Could you check a few things on this drawing? It's one solid part, dimensions in mm from its lowest x, y, z. Give positions to 0.01 mm unless a question says otherwise; leave off trailing zeros. Loops run counter-clockwise (first coordinate to the right, second up) from the corner with the lowest first, then second, coordinate; pieces in that order, holes last. Notation, with made-up numbers: (84.25, 45.25) - (121.25, 45.25) arc R21 cw to (121.25, 55.25) - close; hole circle Ø4 at (28, 56). An arc over 180 degrees is marked (long way). Use a Markdown table: item, result.
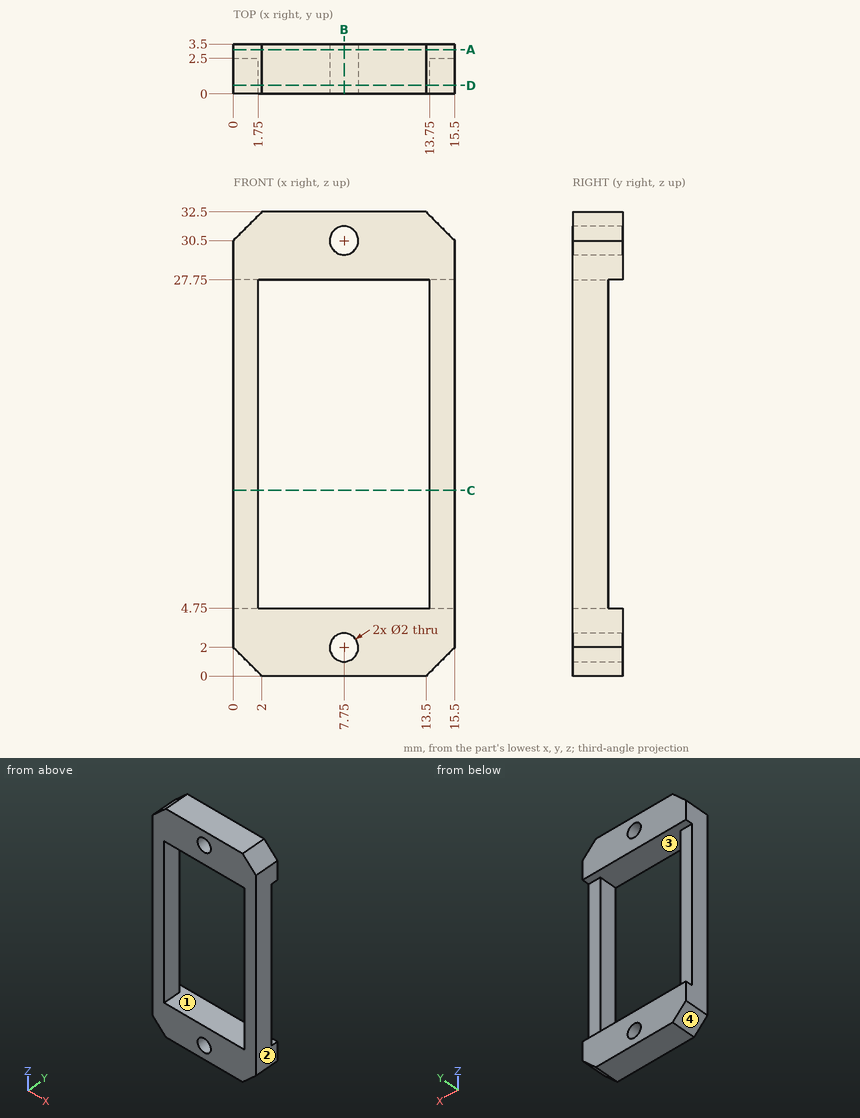
(1) Suppose I cut it at A-A on y = 3.1. Write out the boundary of the cut face in (x, z), plus the area to 3 significant figures.
A:
| item | result |
|---|---|
| outline | (0, 2) - (2, 0) - (13.5, 0) - (15.5, 2) - (15.5, 4.75) - (0, 4.75) - close; (0, 27.75) - (15.5, 27.75) - (15.5, 30.5) - (13.5, 32.5) - (2, 32.5) - (0, 30.5) - close; hole circle Ø2 at (7.75, 2); hole circle Ø2 at (7.75, 30.5) |
| area | 133 mm2 |
(2) We'd pull the mould along Z, two halves only. Please class the marked faces 1, 2, 3 and 4: pulls with the +Z half, pulls with the -Z half, needs draft (parallel to the pull), parting line crosses it, or undercut.
A:
| item | result |
|---|---|
| face 1 | undercut |
| face 2 | needs draft |
| face 3 | undercut |
| face 4 | pulls with the -Z half |
(3) If I drill on line 1 (Z direction, x = 3.75, y = 2.7); line 2 (X direction, y = 2.5, z = 30.5); line 3 (X direction, y = 1.5, z = 20), over which ranges is the centre line in solid material (lowest first)?
A:
| item | result |
|---|---|
| line 1 | 0 to 4.75, 27.75 to 32.5 |
| line 2 | 0 to 6.75, 8.75 to 15.5 |
| line 3 | 0 to 1.75, 13.75 to 15.5 |
(4) Suppose I cut it at C-C on z = 13. Write out the boundary of the cut face in (x, y).
A:
| item | result |
|---|---|
| outline | (0, 0) - (1.75, 0) - (1.75, 2.5) - (0, 2.5) - close; (13.75, 0) - (15.5, 0) - (15.5, 2.5) - (13.75, 2.5) - close |
(5) Will this pin go through, and if not, where does the flat tip stop? pin 1 (0.5 mm diameter, centred on x = 14.5, z = 20.5, fed in from +Y).
A:
| item | result |
|---|---|
| pin 1 | y = 2.5 |
(6) Suppose I cut it at D-D on y = 0.6. Write out the boundary of the cut face in (x, z), plus the area to 3 significant figures.
A:
| item | result |
|---|---|
| outline | (0, 2) - (2, 0) - (13.5, 0) - (15.5, 2) - (15.5, 30.5) - (13.5, 32.5) - (2, 32.5) - (0, 30.5) - close; hole (1.75, 4.75) - (13.75, 4.75) - (13.75, 27.75) - (1.75, 27.75) - close; hole circle Ø2 at (7.75, 2); hole circle Ø2 at (7.75, 30.5) |
| area | 213 mm2 |
(7) Suppose I cut it at B-B on x = 7.75. Write out the boundary of the cut face in (y, z), plus the area to 4 significant figures.
A:
| item | result |
|---|---|
| outline | (0, 0) - (3.5, 0) - (3.5, 1) - (0, 1) - close; (0, 3) - (3.5, 3) - (3.5, 4.75) - (0, 4.75) - close; (0, 27.75) - (3.5, 27.75) - (3.5, 29.5) - (0, 29.5) - close; (0, 31.5) - (3.5, 31.5) - (3.5, 32.5) - (0, 32.5) - close |
| area | 19.25 mm2 |
